Work out the finished part from the listing and answer in its coordinate system (mm). A direction names the side the tool comes from. Coordinates: 2 decimals unless noted, no trailing zeros. Loops run counter-clockwise (first coordinate to the right, second up) from the corner with the lowest first, then second, coordinate; pieces in that order, holes last. Notation, with made-up numbers: (87.5, 71.25) -> (134.5, 71.25) arc R24 cw to (134.5, 90.25) -> close; hole circle Ø8 at (73, 65). An arc over 180 degrees is marked (long way). Use a Markdown table: item, result.
from build123d import *

# Parameters (mm, degrees)
F0_R     = 101.6
F1_DEPTH = 50.8
F2_R     = 25.39999
F3_R     = 16.5014152295
F4_DEPTH = 50.801
F5_DEPTH = 6.35
F6_DEPTH = 6.35


# Not quite as in the source:
# - a fillet or chamfer is up to 0.001 mm smaller than in the source, because OpenCascade refuses the exact size


with BuildPart() as f1:
    # F0 (on Front) → F1 (new body)
    with BuildSketch(Plane.XZ):
        Circle(F0_R)
    extrude(amount=F1_DEPTH)

    # F2 (radius 25.4 in the source; OpenCascade refuses exactly that, so slightly less here)
    f2_edges = [f1.edges().sort_by_distance(p)[0] for p in [
        (-101.6, -50.8, 0),
        (-101.6, 0, 0),
    ]]
    fillet(f2_edges, radius=F2_R)

    # F3 (on face) → F4 (cut, through all)
    with BuildSketch(Plane.XZ.offset(50.8)):
        Circle(F3_R)
    extrude(amount=-F4_DEPTH, mode=Mode.SUBTRACT)

    # F5 (cut): a face of the model
    f5_faces = [f1.faces().sort_by_distance(p)[0] for p in [
        (-74.0447482481, -50.8, 0),
    ]]
    extrude(f5_faces, amount=-F5_DEPTH, mode=Mode.SUBTRACT)

    # F6 (cut): a face of the model
    f6_faces = [f1.faces().sort_by_distance(p)[0] for p in [
        (-74.0447482481, 0, 0),
    ]]
    extrude(f6_faces, amount=-F6_DEPTH, mode=Mode.SUBTRACT)


solid = f1.part
Q1. Section C-C on y = -32.5 is taken. Determine the outline of the cut face in (x, z) (1 decimal).
Solved:
| item | result |
|---|---|
| outline | circle Ø201.2 at (0, 0); hole circle Ø33 at (0, 0) |
Q2. Consider line 1 (Z direction, x = 0, y = -26.5); line 2 (Y direction, x = -10.5, z = -25.5); line 3 (Z direction, x = -3, y = -6). Determine where each line is inside the solid, lowest interval first. Write a range as [from, to].
Solved:
| item | result |
|---|---|
| line 1 | [-101.58, -16.5], [16.5, 101.58] |
| line 2 | [-44.45, -6.35] |
| line 3 | [-92.55, -76.14], [76.14, 92.55] |
Q3. Given pin 1 Ø2 at (x, y) = (-47, -14) entering from +Z; pin 2 Ø1.5 at (x, z) = (36.5, 58) entering from +Y; pin 3 Ø2 at (y, z) = (-39.5, 40) entering from -X, each flat-ended and moving along its own axis, determine where each tip first touches the part or whether it passes through.
Solved:
| item | result |
|---|---|
| pin 1 | z = 87.78 |
| pin 2 | y = -6.35 |
| pin 3 | x = -89.56 |
Q4. For faces 1 (the cylindrical face through (-13.095, -25.667, -10.041)), 2 (the flat face through (-1, -6.35, 18)), 3 (the cylindrical face through (-16.519, -47.669, -74.388)), determine the directions among +Z, -Z, +X, -X, +Y, -Y from which every point of the face is accessible in a straight line to the end or side of a thin tool.
Solved:
| item | result |
|---|---|
| face 1 | +Y, -Y |
| face 2 | +Y |
| face 3 | -Y |
